Part model, mm, in its own coordinate system. A direction names the side the tool comes from. Round coordinates to 2 decimals unless told otherwise and drop trailing zeros. Loops run counter-clockwise (first coordinate to the right, second up) from the corner with the lowest first, then second, coordinate; pieces in that order, holes last. Notation, with made-up numbers: M -34,-25.75 L -24,-25.75 A23 ccw -24,5.25 Z; hole C 13.5,65 d8. An arc over 180 degrees is marked long. Put each result on its own line as item: value. Start each with the question number.
1) Drop a flat-ended pin along its axis: pin 1 Ø0.6 at (x, z) = (-10, -7) entering from -Y. Give the stop position or say it passes through.
2) Slice it at B-B on x = -30. Give the cut face in (y, z).
3) Probe line 1 along X through (y, z) = (14.5, -5); line 2 along Z through (x, y) = (-1.5, 1); line 3 along X through (y, z) = (2.75, -12.75). List the from-to ranges inside material, lowest first.
4) Pull direction Z, two halves, no side cores. Call faces 4 (the flat face through (-29, 3, -13)), 5 (the flat face through (-25, 2, -7)), 6 (the flat face through (-13, 15, -8)), 7 (the flat face through (-13, 7, 0)): +Z half, -Z half, draft (parallel to the pull), parting line (faces both ways), or undercut.
5) Slice it at D-D on x = -3.5. Give the cut face in (y, z), then the cut area to 3 significant figures.
6) Which spindle directions (+Z, -Z, +X, -X, +Y, -Y) get a long thin tool onto all of the face, cutting with end or side? Do faces 1 (the flat face through (-5, 6, -2)), 2 (the flat face through (-34, 8, -8)), 3 (the flat face through (0, 9, -7)). Say none if no direction does.
7) Slice it at A-A on y = 4.5. State how many separate pieces and enclosed holes the cut face has, then the cut area to 3 significant figures.
8) Slice it at C-C on y = 14. Give the cut face in (x, z), then the cut area to 3 significant figures.
```python
from build123d import *

# Parameters (mm, degrees)
SKETCH1_W           = 6
SKETCH1_H           = 15
BOSS_EXTRUDE1_DEPTH = 15
SKETCH2_W           = 4
SKETCH2_H           = 11
CUT_EXTRUDE1_DEPTH  = 13
SKETCH3_W           = 15
SKETCH3_H           = 4
BOSS_EXTRUDE2_DEPTH = 2
LPATTERN1_COUNT     = 4
LPATTERN1_PITCH     = 8
SKETCH4_W           = 15
SKETCH4_H           = 15
BOSS_EXTRUDE3_DEPTH = 8
SKETCH5_W           = 4
SKETCH5_H           = 11
CUT_EXTRUDE2_DEPTH  = 5.5
SKETCH6_W           = 15
SKETCH6_H           = 15
BOSS_EXTRUDE4_DEPTH = 2
SKETCH7_W           = 36
SKETCH7_H           = 2
CUT_EXTRUDE3_DEPTH  = 2


with BuildPart() as part:
    # Sketch1 → Boss-Extrude1 (new body)
    with BuildSketch(Plane(origin=(0, 0, 0), x_dir=(1, 0, 0), z_dir=(0, 1, 0))):
        with Locations((3, 7.5)):
            Rectangle(SKETCH1_W, SKETCH1_H)
    extrude(amount=BOSS_EXTRUDE1_DEPTH)

    # Sketch2 → Cut-Extrude1 (cut)
    with BuildSketch(Plane.XZ):
        with Locations((3, -7.5)):
            Rectangle(SKETCH2_W, SKETCH2_H)
    extrude(amount=-CUT_EXTRUDE1_DEPTH, mode=Mode.SUBTRACT)

    # Sketch3 → Boss-Extrude2 (add)
    with BuildSketch(Plane.ZY):
        with Locations((-7.5, 2)):
            Rectangle(SKETCH3_W, SKETCH3_H)
    extrude(amount=BOSS_EXTRUDE2_DEPTH)


with BuildPart() as lpattern1_1:
    # LPattern1: pattern copy
    add(part.part.moved(Location(Vector(-1, 0, 0) * (1 * LPATTERN1_PITCH))))


with BuildPart() as lpattern1_2:
    # LPattern1: pattern copy
    add(part.part.moved(Location(Vector(-1, 0, 0) * (2 * LPATTERN1_PITCH))))


with BuildPart() as lpattern1_3:
    # LPattern1: pattern copy
    add(part.part.moved(Location(Vector(-1, 0, 0) * (3 * LPATTERN1_PITCH))))

    # Sketch4 → Boss-Extrude3 (add)
    with BuildSketch(Plane.ZY.offset(26)):
        with Locations((-7.5, 7.5)):
            Rectangle(SKETCH4_W, SKETCH4_H)
    extrude(amount=BOSS_EXTRUDE3_DEPTH)

    # Sketch5 → Cut-Extrude2 (cut)
    with BuildSketch(Plane.XZ):
        with Locations((-29, -7.5)):
            Rectangle(SKETCH5_W, SKETCH5_H)
    extrude(amount=-CUT_EXTRUDE2_DEPTH, mode=Mode.SUBTRACT)


with BuildPart() as lpattern1_1_1:
    add(lpattern1_1.part)

    # Combine1: union LPattern1_2, LPattern1_3, part
    add(lpattern1_2.part)
    add(lpattern1_3.part)
    add(part.part)

    # Sketch6 → Boss-Extrude4 (add)
    with BuildSketch(Plane(origin=(6, 0, 0), x_dir=(0, 0, -1), z_dir=(1, 0, 0))):
        with Locations((7.5, 7.5)):
            Rectangle(SKETCH6_W, SKETCH6_H)
    extrude(amount=BOSS_EXTRUDE4_DEPTH)

    # Sketch7 → Cut-Extrude3 (cut)
    with BuildSketch(Plane.XZ):
        with Locations((-13, -7.5)):
            Rectangle(SKETCH7_W, SKETCH7_H)
    extrude(amount=-CUT_EXTRUDE3_DEPTH, mode=Mode.SUBTRACT)


solid = lpattern1_1_1.part
```
Recorded:
1. pin 1: stops at y = 2
2. outline: M 0,-15 L 15,-15 L 15,0 L 0,0 L 0,-2 L 5.5,-2 L 5.5,-13 L 0,-13 Z
3. line 1: x = -34 to -26, -24 to -18, -16 to -10, -8 to -2, 0 to 8
3. line 2: z = -15 to -8.5, -6.5 to 0
3. line 3: x = -34 to -31, -27 to -23, -19 to -15, -11 to -7, -3 to 1, 5 to 8
4. face 4: undercut
4. face 5: undercut
4. face 6: draft
4. face 7: +Z half
5. outline: M 0,-15 L 15,-15 L 15,0 L 0,0 L 0,-2 L 13,-2 L 13,-13 L 0,-13 Z
5. area: 82.0 mm2
6. face 1: -Y
6. face 2: +Z, -Z, -X, +Y, -Y
6. face 3: +Z, -Z, +Y
7. separate pieces: 5
7. enclosed holes: 5
7. area: 290 mm2
8. outline: M -34,-15 L -26,-15 L -26,0 L -34,0 Z; M -24,-15 L -18,-15 L -18,0 L -24,0 Z; M -16,-15 L -10,-15 L -10,0 L -16,0 Z; M -8,-15 L -2,-15 L -2,0 L -8,0 Z; M 0,-15 L 8,-15 L 8,0 L 0,0 Z
8. area: 510 mm2
